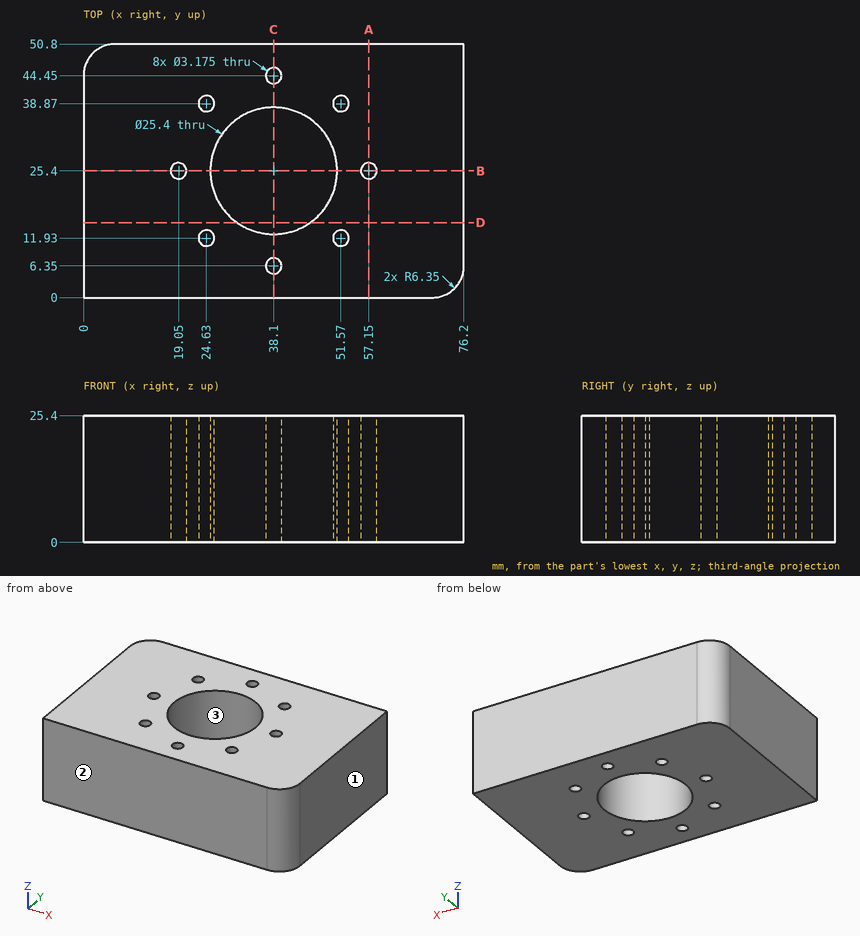
Here's the drawing with two shaded views (mm, measured from the low corner). I have some questions. Coordinates: 2 decimals unless noted, no trailing zeros. Write each loop counter-clockwise with the first axis right and the second up, starting at its lowest first coordinate (ties: lowest second). Pieces come first, ordered by that corner, then holes. Notation, with made-up numbers: (74.25, 71) -> (131.25, 71) arc R12 ccw to (131.25, 93) -> close; hole circle Ø8 at (21.25, 34). An arc over 180 degrees is marked (long way). Use a Markdown table: item, result. Add a question column.
(1) Please list where these lines run through material, in increasing order: line 1 (Y direction, x = 38.1, z = 8.75); line 2 (Y direction, x = 24.5, z = 16.75); line 3 (Y direction, x = 19.05, z = 20).
(2) If we section it at B-B, the plane y = 25.4: Write out the boundary of the cut face in (x, z).
(3) If we section it at A-A, the plane x = 57.15: Write out the boundary of the cut face in (y, z), and give its area (3 significant figures).
(4) We'd pull the mould along X, two halves only. Please class the marked faces 1, 2 and 3: +X half, -X half, draft (parallel to the pull), parting line (faces both ways), or undercut.
(5) If we section it at C-C, the plane x = 38.1: Write out the boundary of the cut face in (y, z).
(6) If we section it at D-D, the plane y = 15: Write out the boundary of the cut face in (x, z).
Outcome:
| question | item | result |
|---|---|---|
| 1 | line 1 | y = 0 to 4.76, 7.94 to 12.7, 38.1 to 42.86, 46.04 to 50.8 |
| 1 | line 2 | y = 0 to 10.35, 13.51 to 37.29, 40.45 to 50.8 |
| 1 | line 3 | y = 0 to 23.81, 26.99 to 50.8 |
| 2 | outline | (0, 0) -> (17.46, 0) -> (17.46, 25.4) -> (0, 25.4) -> close; (20.64, 0) -> (25.4, 0) -> (25.4, 25.4) -> (20.64, 25.4) -> close; (50.8, 0) -> (55.56, 0) -> (55.56, 25.4) -> (50.8, 25.4) -> close; (58.74, 0) -> (76.2, 0) -> (76.2, 25.4) -> (58.74, 25.4) -> close |
| 3 | outline | (0, 0) -> (23.81, 0) -> (23.81, 25.4) -> (0, 25.4) -> close; (26.99, 0) -> (50.8, 0) -> (50.8, 25.4) -> (26.99, 25.4) -> close |
| 3 | area | 1,210 mm^2 |
| 4 | face 1 | +X half |
| 4 | face 2 | draft |
| 4 | face 3 | undercut |
| 5 | outline | (0, 0) -> (4.76, 0) -> (4.76, 25.4) -> (0, 25.4) -> close; (7.94, 0) -> (12.7, 0) -> (12.7, 25.4) -> (7.94, 25.4) -> close; (38.1, 0) -> (42.86, 0) -> (42.86, 25.4) -> (38.1, 25.4) -> close; (46.04, 0) -> (50.8, 0) -> (50.8, 25.4) -> (46.04, 25.4) -> close |
| 6 | outline | (0, 0) -> (30.81, 0) -> (30.81, 25.4) -> (0, 25.4) -> close; (45.39, 0) -> (76.2, 0) -> (76.2, 25.4) -> (45.39, 25.4) -> close |
